```python
from build123d import *

# Parameters (mm, degrees)
BOSS_EXTRUDE1_DEPTH           = 10
SKETCH2_W                     = 10
SKETCH2_H                     = 5.8
BOSS_EXTRUDE2_DEPTH           = 0.8
TAP_DRILL_FOR_M3_5X0_6_TAP1_D = 2.9
CHAMFER1_SIZE                 = 0.379
FILLET1_R                     = 0.2


with BuildPart() as part:
    # Sketch1 → Boss-Extrude1 (new body)
    with BuildSketch(Plane.XY.offset(5)):
        with BuildLine():
            Line((-0.8, -4.771898466), (-0.8, 4.771898466))
            ThreePointArc((-0.8, 4.771898466), (-0.922761052, 4.974218302), (-1.158906761, 4.958765267))
            Line((-1.158906761, 4.958765267), (-4.1, 2.9))
            Line((-4.1, 2.9), (-4.1, -2.9))
            Line((-4.1, -2.9), (-1.158906761, -4.958765267))
            ThreePointArc((-1.158906761, -4.958765267), (-0.922761052, -4.974218302), (-0.8, -4.771898466))
        make_face()
    extrude(amount=-BOSS_EXTRUDE1_DEPTH)

    # Sketch2 → Boss-Extrude2 (add)
    with BuildSketch(Plane(origin=(-0.8, 0, 0), x_dir=(0, 0, -1), z_dir=(1, 0, 0))):
        Rectangle(SKETCH2_W, SKETCH2_H)
    extrude(amount=BOSS_EXTRUDE2_DEPTH)

    # Tap Drill for M3.5x0.6 Tap1 (through all)
    with Locations(Plane(origin=(0, 0, 0), x_dir=(0, 0, -1), z_dir=(1, 0, 0))):
        with Locations((0, 0)):
            Hole(TAP_DRILL_FOR_M3_5X0_6_TAP1_D / 2)

    # Chamfer1
    chamfer1_edges = [part.edges().sort_by_distance(p)[0] for p in [
        (0, 0, -1.45),
        (-4.1, 0, -1.45),
    ]]
    chamfer(chamfer1_edges, length=CHAMFER1_SIZE)

    # Fillet1
    fillet1_edges = [part.edges().sort_by_distance(p)[0] for p in [
        (-4.1, -2.9, 0),
        (-4.1, 2.9, 0),
        (0, 2.9, 0),
        (0, -2.9, 0),
    ]]
    fillet(fillet1_edges, radius=FILLET1_R)


solid = part.part
```
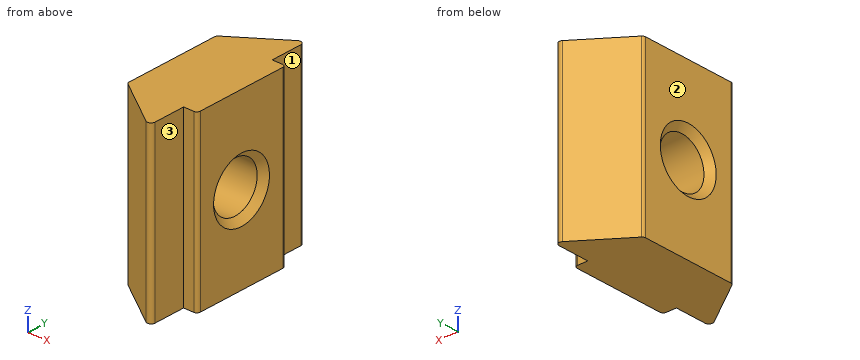
Input: part model. Units: mm. Frame: model coordinates. Face numbers are marked on the shaded views. A direction names the side the tool comes from. Give positions to 0.01 mm unless a question says otherwise; leave off trailing zeros. Order: outer loops, then holes, each group sorted by start corner. A loop starts at its lowest first (then second) coordinate and runs counter-clockwise, first axis right, second up. Notation, with made-up numbers: (-24.5, 30.25) - (8.5, 30.25) arc R29 ccw to (8.5, 60.25) - close; hole circle Ø5 at (-7, 51.25). An arc over 180 degrees is marked (long way). Put each result on its own line as item: value.
Item 1: Section query C-C, the plane x = -3.4. Return loops of the section in (y, z), then the cut area to 3 significant figures.
Found:
outline: (-3.39, -5) - (3.39, -5) - (3.39, 5) - (-3.39, 5) - close; hole circle Ø2.9 at (0, 0)
area: 61.2 mm^2
Item 2: Ray query, L1, parallel to Y at x = -2, z = 0; L2, parallel to Y at x = -1.5, z = 0; L3, parallel to Y at x = -0.25, z = -1.75. Return the intervals inside material, ascending. Write a range as from..to.
Found:
L1: y = -4.37..-1.45, 1.45..4.37
L2: y = -4.72..-1.45, 1.45..4.72
L3: y = -2.9..2.9
Item 3: Access query for the marked faces 1, 2 and 3. Directions: +Z, -Z, +X, -X, +Y, -Y. A direction counts if a zero-diameter tool reaches every point of the face in a straight line with its end or side. Return the directions, or none.
Found:
face 1: +Z, -Z, +X, +Y
face 2: +Z, -Z, -X, +Y, -Y
face 3: +Z, -Z, +X, -Y
Item 4: Section query B-B, the plane z = 0. Return loops of the section in (x, y), then the cut area to 3 significant figures.
Found:
outline: (-4.1, -2.8) arc R0.2 ccw to (-4.01, -2.96) - (-1.16, -4.96) arc R0.23 ccw to (-0.8, -4.77) - (-0.8, -2.9) - (-0.2, -2.9) arc R0.2 ccw to (0, -2.7) - (0, -1.83) - (-0.38, -1.45) - (-3.72, -1.45) - (-4.1, -1.83) - close; (-4.1, 1.83) - (-3.72, 1.45) - (-0.38, 1.45) - (0, 1.83) - (0, 2.7) arc R0.2 ccw to (-0.2, 2.9) - (-0.8, 2.9) - (-0.8, 4.77) arc R0.23 ccw to (-1.16, 4.96) - (-4.01, 2.96) arc R0.2 ccw to (-4.1, 2.8) - close
area: 19.1 mm^2
Item 5: Section query D-D, the plane z = 3.75. Return loops of the section in (x, y), then the cut area to 3 significant figures.
Found:
outline: (-4.1, -2.8) arc R0.2 ccw to (-4.01, -2.96) - (-1.16, -4.96) arc R0.23 ccw to (-0.8, -4.77) - (-0.8, -2.9) - (-0.2, -2.9) arc R0.2 ccw to (0, -2.7) - (0, 2.7) arc R0.2 ccw to (-0.2, 2.9) - (-0.8, 2.9) - (-0.8, 4.77) arc R0.23 ccw to (-1.16, 4.96) - (-4.01, 2.96) arc R0.2 ccw to (-4.1, 2.8) - close
area: 31.3 mm^2
Item 6: Contact query for flat-ended pins moving along their axis: pin 1 (1.5 mm diameter, centred on y = 4, z = 0.5, fed in from +X); pin 2 (3.5 mm diameter, centred on y = 0, z = 0, fed in from +X). Output: stop coordinate, or through.
Found:
pin 1: stops at x = -0.8
pin 2: stops at x = -0.08
Item 7: Section query A-A, the plane y = 0. Return loops of the section in (x, z).
Found:
outline: (-4.1, -5) - (0, -5) - (0, -1.83) - (-0.38, -1.45) - (-3.72, -1.45) - (-4.1, -1.83) - close; (-4.1, 1.83) - (-3.72, 1.45) - (-0.38, 1.45) - (0, 1.83) - (0, 5) - (-4.1, 5) - close
